```python
from build123d import *

# Parameters (mm, degrees)
POCKET_DEPTH         = 35
SKETCH003_R          = 10
SKETCH003_R_2        = 7
POCKET001_DEPTH      = 30.001
POCKET001_DEPTH_BACK = -30.001
POCKET002_DEPTH      = 5


with BuildPart() as part:
    # Sketch → Revolution (revolve)
    with BuildSketch(Plane.YZ):
        Polygon((-25, 20), (-85, 20), (-85, 0), (95, 0), (95, 24), (25, 24), (25, 30), (-25, 30), align=None)
    revolve(axis=Axis((0, 0, 0), (0, 1, 0)))

    # Sketch002 (on Face2 of Revolution) → Pocket (cut)
    with BuildSketch(Plane(origin=(0, -85, 0), x_dir=(0, 0, -1), z_dir=(0, -1, 0))):
        with BuildLine():
            Line((-12, -16), (-12, 16))
            ThreePointArc((-12, 16), (-20, 0), (-12, -16))
        make_face()
    extrude(amount=-POCKET_DEPTH, mode=Mode.SUBTRACT)

    # Sketch003 → Pocket001 (cut, two sides)
    with BuildSketch(Plane.XY) as pocket001_sk:
        Circle(SKETCH003_R)
        with Locations((0, -70)):
            Circle(SKETCH003_R_2)
    extrude(amount=-POCKET001_DEPTH, mode=Mode.SUBTRACT)
    extrude(pocket001_sk.sketch, amount=-POCKET001_DEPTH_BACK, mode=Mode.SUBTRACT)

    # Sketch004 (on DatumPlane) → Pocket002 (cut)
    with BuildSketch(Plane.XY.offset(19)):
        with BuildLine():
            ThreePointArc((7, 71), (0, 78), (-7, 71))
            Line((-7, 71), (-7, 49))
            ThreePointArc((-7, 49), (0, 42), (7, 49))
            Line((7, 71), (7, 49))
        make_face()
    extrude(amount=POCKET002_DEPTH, mode=Mode.SUBTRACT)


solid = part.part
```
Design review of the part built by this model. Coordinates are the model's own, in mm. A direction names the side the tool comes from. Round coordinates to 2 decimals unless told otherwise and drop trailing zeros. Order: outer loops, then holes, each group sorted by start corner. A loop starts at its lowest first (then second) coordinate and runs counter-clockwise, first axis right, second up. Notation, with made-up numbers: (-10.5, -39) - (15.5, -39) arc R22 cw to (15.5, -17) - close; hole circle Ø6 at (23, 78). An arc over 180 degrees is marked (long way). Return JSON: item names as keys, results as strings.
Q1. Consider section B-B on z = 10. Write out the cut boundary in (x, y), plus the area to 3 significant figures.
Computed values:
{"outline": "(-28.28, -25) - (-17.32, -25) - (-17.32, -85) - (17.32, -85) - (17.32, -25) - (28.28, -25) - (28.28, 25) - (21.82, 25) - (21.82, 95) - (-21.82, 95) - (-21.82, 25) - (-28.28, 25) - close; hole circle Ø20 at (0, 0); hole circle Ø14 at (0, -70)", "area": "7,490 mm2"}
Q2. For pin 1 Ø5 at (x, y) = (17.5, 33) entering from +Z (3 decimals); pin 2 Ø4 at (x, y) = (13.5, 38.5) entering from -Z; pin 3 Ø12 at (x, y) = (13.5, -17) entering from -Z; pin 4 Ø9 at (x, z) = (-5.5, 14.5) entering from -Y, all flat-tipped, find the tip position at first contact; note any pin that passes through.
Computed values:
{"pin 1": "stops at z = 18.735", "pin 2": "stops at z = -21.07", "pin 3": "stops at z = -29.05", "pin 4": "stops at y = -85"}
Q3. The part is to be moulded in two halves that separate along Y. For faces 6 (the flat face through (20.1, 25, 13.5)), 7 (the cylindrical face through (0, 78, 21)), 8 (the cylindrical face through (0, 42, 21)), 9 (the flat face through (0, -50, 15)), say which applies: pulls with the +Y half, pulls with the -Y half, needs draft (parallel to the pull), parting line crosses it, or undercut.
Computed values:
{"face 6": "pulls with the +Y half", "face 7": "undercut", "face 8": "undercut", "face 9": "pulls with the -Y half"}
Q4. Consider section C-C on y = -70. Write out the cut boundary in (x, z) (3 decimals), plus the area to 3 significant figures.
Computed values:
{"outline": "(-16, 12) arc R20 ccw to (-7, -18.735) - (-7, 12) - close; (7, -18.735) arc R20 ccw to (16, 12) - (7, 12) - close", "area": "636 mm2"}
Q5. Wall thickness on L1, parallel to Y at x = 0, z = -17.5; L2, parallel to X at y = -70, z = 1; L3, parallel to Y at x = -4, z = -8.5: over which ranges is each line inside the solid? List them lowest first. Write a range as [from, to].
Computed values:
{"L1": "y = [-85, -77], [-63, -10], [10, 95]", "L2": "x = [-19.97, -7], [7, 19.97]", "L3": "y = [-85, -75.74], [-64.26, -9.17], [9.17, 95]"}
Q6. Consider section A-A on x = 0. Write out the cut boundary in (y, z).
Computed values:
{"outline": "(-85, -20) - (-77, -20) - (-77, 12) - (-85, 12) - close; (-63, -20) - (-25, -20) - (-25, -30) - (-10, -30) - (-10, 30) - (-25, 30) - (-25, 20) - (-50, 20) - (-50, 12) - (-63, 12) - close; (10, -30) - (25, -30) - (25, -24) - (95, -24) - (95, 24) - (78, 24) - (78, 19) - (42, 19) - (42, 24) - (25, 24) - (25, 30) - (10, 30) - close"}
Q7. Consider section D-D on y = -36. Write out the cut boundary in (x, z), plus the area to 3 significant figures.
Computed values:
{"outline": "circle Ø40 at (0, 0)", "area": "1,260 mm2"}
Q8. Machinability: for faces 1 (the flat face through (-7, 60, 21)), 2 (the flat face through (0, -85, -4)), 3 (the cylindrical face through (1.055, 59.51, -23.977)), 4 (the cylindrical face through (0.88, -55.42, -19.98)), 5 (the flat face through (-4, -64, 12)), which of the approach directions +Z, -Z, +X, -X, +Y, -Y give a long, thin tool a straight path to every point of the face, cutting with its end or side? Answer none if there is none.
Computed values:
{"face 1": "+Z", "face 2": "+Z, -Z, +X, -X, -Y", "face 3": "+Y", "face 4": "-Y", "face 5": "+Z, +X, -X, -Y"}
